Here's how the part is built. I have some questions about the finished solid (model axes, mm). Face numbers are marked on the shaded views. A direction names the side the tool comes from. Give positions to 0.01 mm unless a question says otherwise; leave off trailing zeros. Write each loop counter-clockwise with the first axis right and the second up, starting at its lowest first coordinate (ties: lowest second). Pieces come first, ordered by that corner, then holes. Notation, with made-up numbers: (-3, -28) -> (16, -28) arc R12 ccw to (16, -6) -> close; hole circle Ø9 at (81.25, 56.25). An arc over 180 degrees is marked (long way). Return JSON: item names as keys, results as strings.
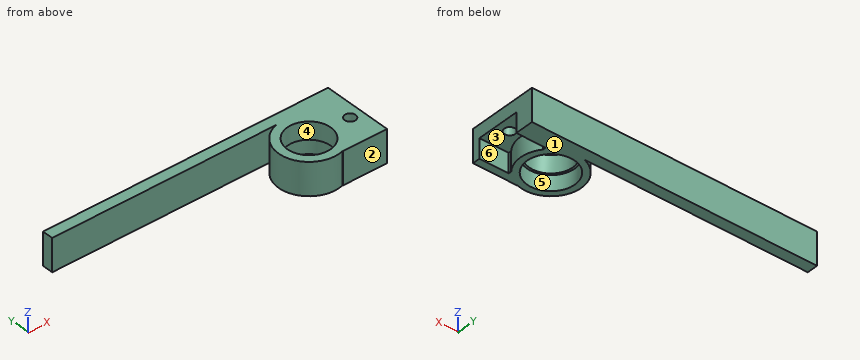
from build123d import *

# Parameters (mm, degrees)
SKETCH_1_W          = 40
SKETCH_1_H          = 20
EXTRUDE_1_DEPTH     = 6
SKETCH_2_R          = 2.5
CUT_EXTRUDE_1_DEPTH = 24.151673806
EXTRUDE_START       = -15
EXTRUDE_2_OUTLINE_R = 11
EXTRUDE_2_DEPTH     = 15
EXTRUDE_START_2     = -8
SKETCH_5_R          = 11
SKETCH_5_R_2        = 10
EXTRUDE_3_DEPTH     = 8
SKETCH_8_W          = 15
SKETCH_8_H          = 5
EXTRUDE_4_DEPTH     = 500
SKETCH_9_W          = 4.037306924
SKETCH_9_H          = 3.364422437
EXTRUDE_5_DEPTH     = 15
SKETCH_10_W         = 26.5
SKETCH_10_H         = 32
CUT_EXTRUDE_2_DEPTH = 481.59052217
SKETCH_12_W         = 363.719511947
SKETCH_12_H         = 27.53578134
CUT_EXTRUDE_3_DEPTH = 482.183177179


# Read off the part's stored shape, not the designer's step: 凸台-拉伸2
with BuildPart() as part:
    # 草图1 → 凸台-拉伸1 (new body)
    with BuildSketch(Plane.XY):
        Rectangle(SKETCH_1_W, SKETCH_1_H)
    extrude(amount=EXTRUDE_1_DEPTH)

    # 草图2 → 切除-拉伸1 (cut, through all)
    with BuildSketch(Plane.XY.offset(6)):
        with Locations((10, 0)):
            Circle(SKETCH_2_R)
        with Locations((-1, 0)):
            Circle(SKETCH_2_R)
        with Locations((-12, 0)):
            Circle(SKETCH_2_R)
    extrude(amount=-CUT_EXTRUDE_1_DEPTH, mode=Mode.SUBTRACT)

    # 凸台-拉伸2 outline → 凸台-拉伸2 (add)
    with BuildSketch(Plane.XY.offset(6).offset(EXTRUDE_START)):
        with BuildLine():
            Line((20, 10), (20, 13.5))
            Line((20, 13.5), (-26.893967141, 13.5))
            Line((-26.893967141, 13.5), (-26.893967141, 13.384337644))
            ThreePointArc((-26.893967141, 13.384337644), (-45, 0), (-26.893967141, -13.384337644))
            Line((-26.893967141, -13.384337644), (-26.893967141, -13.5))
            Line((-26.893967141, -13.5), (20, -13.5))
            Line((20, -13.5), (20, -10))
            Line((20, -10), (-20, -10))
            Line((-20, -10), (-20, -8.660254038))
            ThreePointArc((-20, -8.660254038), (-17, 0), (-20, 8.660254038))
            Line((-20, 8.660254038), (-20, 10))
            Line((-20, 10), (20, 10))
        make_face()
        with Locations((-31, 0)):
            Circle(EXTRUDE_2_OUTLINE_R, mode=Mode.SUBTRACT)
    extrude(amount=EXTRUDE_2_DEPTH)

    # 草图5 → 凸台-拉伸3 (add)
    with BuildSketch(Plane.XY.offset(6).offset(EXTRUDE_START_2)):
        with Locations((-31, 0)):
            Circle(SKETCH_5_R)
        with Locations((-31, 0)):
            Circle(SKETCH_5_R_2, mode=Mode.SUBTRACT)
    extrude(amount=EXTRUDE_3_DEPTH)

    # 草图8 → 凸台-拉伸4 (add)
    with BuildSketch(Plane(origin=(20, 0, 0), x_dir=(0, 0, -1), z_dir=(1, 0, 0))):
        with Locations((1.5, 16)):
            Rectangle(SKETCH_8_W, SKETCH_8_H)
    extrude(amount=-EXTRUDE_4_DEPTH)

    # 草图9 → 凸台-拉伸5 (add, through all)
    with BuildSketch(Plane(origin=(0, 0, -9), x_dir=(-1, 0, 0), z_dir=(0, 0, -1))):
        with Locations((26.475334378, 14.151164675)):
            Rectangle(SKETCH_9_W, SKETCH_9_H)
    extrude(amount=-EXTRUDE_5_DEPTH)

    # 草图10 → 切除-拉伸2 (cut, through all)
    with BuildSketch(Plane.XY.offset(6)):
        with Locations((6.75, 2.5)):
            Rectangle(SKETCH_10_W, SKETCH_10_H)
    extrude(amount=-CUT_EXTRUDE_2_DEPTH, mode=Mode.SUBTRACT)

    # 草图12 → 切除-拉伸3 (cut, through all)
    with BuildSketch(Plane(origin=(0, 18.5, 0), x_dir=(1, 0, 0), z_dir=(0, 1, 0))):
        with Locations((-319.875382276, 7.753964269)):
            Rectangle(SKETCH_12_W, SKETCH_12_H)
    extrude(amount=-CUT_EXTRUDE_3_DEPTH, mode=Mode.SUBTRACT)


solid = part.part
1. Suppose I cut it at A-A, the plane y = 0. List the corners of the cut face in (x, z) for me, and give its area (3 significant figures).
Taken from the geometry:
{"outline": "(-45, -9) -> (-42, -9) -> (-42, -2) -> (-41, -2) -> (-41, 6) -> (-45, 6) -> close; (-21, -2) -> (-20, -2) -> (-20, -9) -> (-17, -9) -> (-17, 0) -> (-14.5, 0) -> (-14.5, 6) -> (-21, 6) -> close; (-9.5, 0) -> (-6.5, 0) -> (-6.5, 6) -> (-9.5, 6) -> close", "area": "139 mm²"}
2. Suppose I cut it at D-D, the plane z = 4.25. List the corners of the cut face in (x, y) for me.
Taken from the geometry:
{"outline": "(-138.02, 13.5) -> (-34.71, 13.5) arc R14 ccw (long way) to (-26.89, -13.38) -> (-26.89, -13.5) -> (-6.5, -13.5) -> (-6.5, 18.5) -> (-138.02, 18.5) -> close; hole circle Ø20 at (-31, 0); hole circle Ø5 at (-12, 0)"}
3. For pin 1 Ø1 at (y, z) = (-6.5, 0) entering from -X; pin 2 Ø1 at (x, z) = (-43, -0.5) entering from -Y; pin 3 Ø4.5 at (x, z) = (-12, 1.5) entering from -Y, each with a flat end and sliding along its axis, tell me the tip position at first contact or that it passes through.
Taken from the geometry:
{"pin 1": "stops at x = -43.65", "pin 2": "stops at y = -7.98", "pin 3": "stops at y = -13.5"}
4. If we mould it in two halves opening along Y, with no side actions, what happens to the marked faces 1, 2 and 3? For each: released by +Y, released by -Y, zero draft, split by the parting line, or undercut.
Taken from the geometry:
{"face 1": "zero draft", "face 2": "released by -Y", "face 3": "undercut"}
5. If I drill on line 1 (Y direction, x = -31, z = -4.5); line 2 (Y direction, x = -31, z = 2.5); line 3 (Y direction, x = -39, z = -1.75), over which ranges is the centre line in solid material (lowest first)? Write a range as [from, to].
Taken from the geometry:
{"line 1": "y = [-14, -11], [11, 18.5]", "line 2": "y = [-14, -10], [10, 18.5]", "line 3": "y = [-11.49, -6], [6, 11.49], [13.5, 18.5]"}
6. Which directions (+Z, -Z, +X, -X, +Y, -Y) give clear straight access to the entire face, cutting with the end or side of a thin tool? Please do the marked faces 4, 5 and 6.
Taken from the geometry:
{"face 4": "+Z, -Z", "face 5": "-Z", "face 6": "-Z, +X"}
7. Suppose I cut it at B-B, the plane x = -31. List the corners of the cut face in (y, z) for me.
Taken from the geometry:
{"outline": "(-14, -9) -> (-11, -9) -> (-11, -2) -> (-10, -2) -> (-10, 6) -> (-14, 6) -> close; (10, -2) -> (11, -2) -> (11, -9) -> (18.5, -9) -> (18.5, 6) -> (10, 6) -> close"}
8. Suppose I cut it at C-C, the plane z = -6.5. List the corners of the cut face in (x, y) for me.
Taken from the geometry:
{"outline": "(-138.02, 13.5) -> (-34.71, 13.5) arc R14 ccw (long way) to (-26.89, -13.38) -> (-26.89, -13.5) -> (-6.5, -13.5) -> (-6.5, -10) -> (-20, -10) -> (-20, -8.66) arc R14 ccw to (-20, 8.66) -> (-20, 10) -> (-6.5, 10) -> (-6.5, 18.5) -> (-138.02, 18.5) -> close; hole circle Ø22 at (-31, 0)"}
